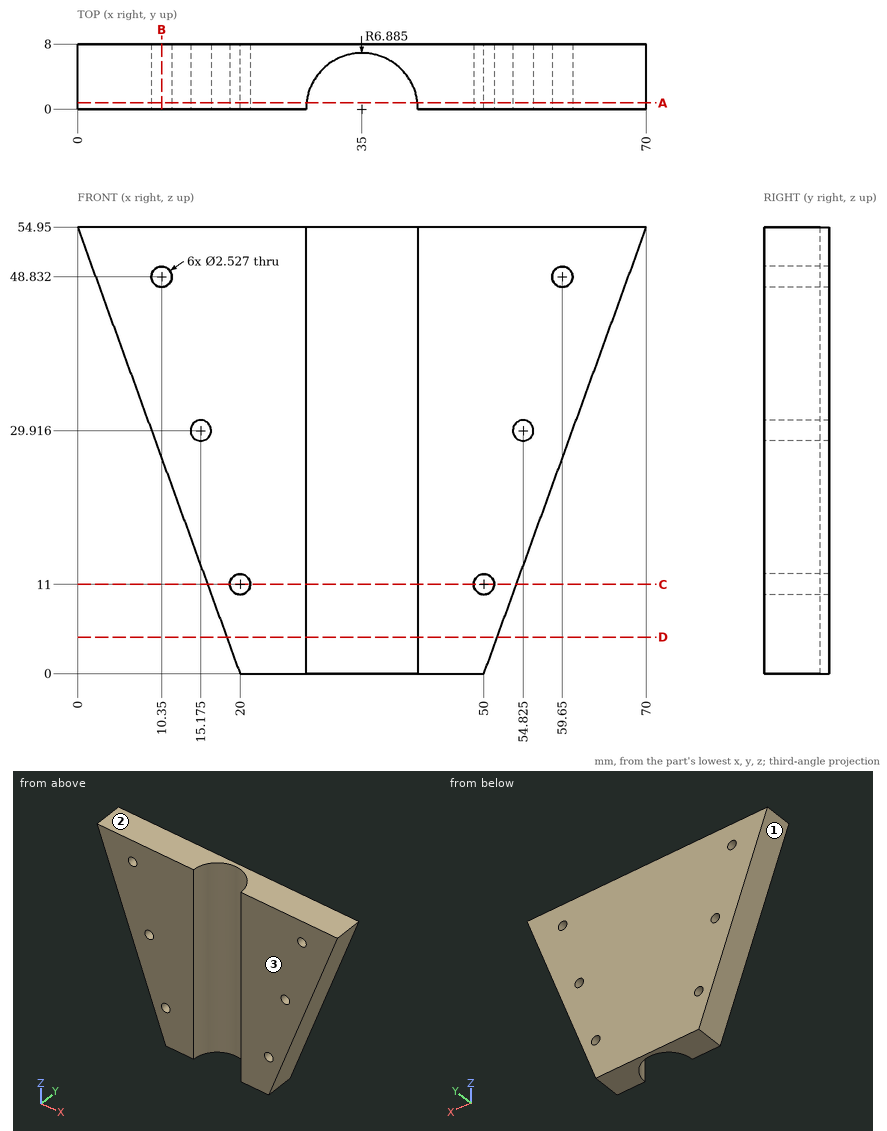
Answer from the drawing. Dimensions are ordinates in mm from the lowest x, y and z of the part. Give positions to 0.01 mm unless a question says otherwise; leave off trailing zeros. Loops run counter-clockwise (first coordinate to the right, second up) from the corner with the lowest first, then second, coordinate; pieces in that order, holes last.
Item 1: A cutting plane is placed at D-D (z = 4.5). Give the vertices of the cut face in (x, y) (1 decimal), then the cut area to 3 significant figures.
Derived:
outline: (18.4, 0) - (28.1, 0) arc R6.9 cw to (41.9, 0) - (51.6, 0) - (51.6, 8) - (18.4, 8) - close
area: 192 mm2
Item 2: Determine the mould class of the marked faces 1, 2 and 3 for opening direction Z: +Z half, -Z half, draft (parallel to the pull), parting line (faces both ways), or undercut.
Derived:
face 1: -Z half
face 2: +Z half
face 3: draft
Item 3: Each of these flat-tipped pins is pushed along its axis until it touches: pin 1 Ø10 at (x, z) = (20.5, 8) entering from -Y; pin 2 Ø1.5 at (y, z) = (2.5, 8) entering from +X (1 decimal); pin 3 Ø4 at (y, z) = (2, 9) entering from +X. Where does it stop, or does it pass through?
Derived:
pin 1: stops at y = 0
pin 2: stops at x = 53.2
pin 3: stops at x = 54
Item 4: A cutting plane is placed at A-A (y = 0.75). Give the number of separate pieces and of enclosed holes in the cut face.
Derived:
separate pieces: 2
enclosed holes: 6
Item 5: Find the intervals of material crossed by line 1 along X through (y, z) = (1.5, 49.5) (1 decimal); line 2 along X through (y, z) = (3.5, 11) (1 decimal); line 3 along X through (y, z) = (4, 43.5) (1 decimal), in increasing order.
Derived:
line 1: x = 2 to 9.3, 11.4 to 28.3, 41.7 to 58.6, 60.7 to 68
line 2: x = 16 to 18.7, 21.3 to 29.1, 40.9 to 48.7, 51.3 to 54
line 3: x = 4.2 to 29.4, 40.6 to 65.8
Item 6: A cutting plane is placed at C-C (z = 11). Give the vertices of the cut face in (x, y) (1 decimal), then the cut area to 3 significant figures.
Derived:
outline: (16, 0) - (18.7, 0) - (18.7, 8) - (16, 8) - close; (21.3, 0) - (28.1, 0) arc R6.9 cw to (41.9, 0) - (48.7, 0) - (48.7, 8) - (21.3, 8) - close; (51.3, 0) - (54, 0) - (54, 8) - (51.3, 8) - close
area: 189 mm2
Item 7: A cutting plane is placed at B-B (x = 10.35). Give the vertices of the cut face in (y, z).
Derived:
outline: (0, 26.51) - (8, 26.51) - (8, 47.57) - (0, 47.57) - close; (0, 50.1) - (8, 50.1) - (8, 54.95) - (0, 54.95) - close
